Build history of the part. All positions in model axes, mm. Coordinates: 2 decimals unless noted, no trailing zeros. Order: outer loops, then holes, each group sorted by start corner. A loop starts at its lowest first (then second) coordinate and runs counter-clockwise, first axis right, second up. Notation, with made-up numbers: M 51.25,-25.75 L 57.25,-25.75 A21 cw 57.25,-12.75 Z; hole C -2,-15 d9. An arc over 180 degrees is marked long. Use a Markdown table: item, result. Add a question column.
from build123d import *

# Parameters (mm, degrees)
SKETCH1_R             = 5
BOSS_EXTRUDE1_DEPTH   = 10
BOSS_EXTRUDE1_2_DEPTH = 10
BOSS_EXTRUDE2_START   = 4
SKETCH1_3_W           = 162
SKETCH1_3_H           = 50
SKETCH1_3_W_2         = 154
SKETCH1_3_H_2         = 42
SKETCH1_3_R           = 5
BOSS_EXTRUDE2_DEPTH   = 4
SKETCH1_4_W           = 162
SKETCH1_4_H           = 50
SKETCH1_4_W_2         = 154
SKETCH1_4_H_2         = 42
BOSS_EXTRUDE3_DEPTH   = 96
FILLET1_R             = 4
SKETCH2_W             = 162
SKETCH2_H             = 50
SKETCH2_W_2           = 154
SKETCH2_H_2           = 42
BOSS_EXTRUDE4_DEPTH   = 5
SKETCH2_2_W           = 162
SKETCH2_2_H           = 50
SKETCH2_2_W_2         = 154
SKETCH2_2_H_2         = 42
BOSS_EXTRUDE5_DEPTH   = 5
SKETCH3_R             = 5
CUT_EXTRUDE1_DEPTH    = 10
SKETCH4_W             = 162
SKETCH4_H             = 50
BOSS_EXTRUDE6_DEPTH   = 10


with BuildPart() as part:
    # Sketch1 → Boss-Extrude1 (new body)
    with BuildSketch(Plane(origin=(0, 0, 0), x_dir=(1, 0, 0), z_dir=(0, 1, 0))):
        with Locations(Location((-57, 8.550438596, 0), (0, 0, 270))):
            Circle(SKETCH1_R)
    extrude(amount=-BOSS_EXTRUDE1_DEPTH)



with BuildPart() as body_2:
    # Sketch1 → Boss-Extrude1 2 (new body)
    with BuildSketch(Plane(origin=(0, 0, 0), x_dir=(1, 0, 0), z_dir=(0, 1, 0))):
        with Locations(Location((57, 8.550438596, 0), (0, 0, 270))):
            Circle(SKETCH1_R)
    extrude(amount=-BOSS_EXTRUDE1_2_DEPTH)


with BuildPart() as part_1:
    add(part.part)

    add(body_2.part)  # Boss-Extrude2 merges body 2
    # Sketch1_3 → Boss-Extrude2 (add)
    # profile 1 of 4: a face of its own
    with BuildSketch(Plane(origin=(0, 0, 0), x_dir=(1, 0, 0), z_dir=(0, 1, 0)).offset(BOSS_EXTRUDE2_START)):
        with Locations((0, 8.550438596)):
            Rectangle(SKETCH1_3_W, SKETCH1_3_H)
        with Locations((0, 8.550438596)):
            Rectangle(SKETCH1_3_W_2, SKETCH1_3_H_2, mode=Mode.SUBTRACT)
    # profile 2 of 4: a face of its own
    with BuildSketch(Plane(origin=(0, 0, 0), x_dir=(1, 0, 0), z_dir=(0, 1, 0)).offset(BOSS_EXTRUDE2_START)):
        with Locations((0, 8.550438596)):
            Rectangle(SKETCH1_3_W_2, SKETCH1_3_H_2)
        with Locations(Location((57, 8.550438596, 0), (0, 0, 270))):
            Circle(SKETCH1_3_R, mode=Mode.SUBTRACT)
        with Locations(Location((-57, 8.550438596, 0), (0, 0, 270))):
            Circle(SKETCH1_3_R, mode=Mode.SUBTRACT)
    # profile 3 of 4: a face of its own
    with BuildSketch(Plane(origin=(0, 0, 0), x_dir=(1, 0, 0), z_dir=(0, 1, 0)).offset(BOSS_EXTRUDE2_START)):
        with Locations(Location((-57, 8.550438596, 0), (0, 0, 270))):
            Circle(SKETCH1_3_R)
    # profile 4 of 4: a face of its own
    with BuildSketch(Plane(origin=(0, 0, 0), x_dir=(1, 0, 0), z_dir=(0, 1, 0)).offset(BOSS_EXTRUDE2_START)):
        with Locations(Location((57, 8.550438596, 0), (0, 0, 270))):
            Circle(SKETCH1_3_R)
    extrude(amount=-BOSS_EXTRUDE2_DEPTH)

    # Sketch1_4 → Boss-Extrude3 (add)
    with BuildSketch(Plane(origin=(0, 0, 0), x_dir=(1, 0, 0), z_dir=(0, 1, 0))):
        with Locations((0, 8.550438596)):
            Rectangle(SKETCH1_4_W, SKETCH1_4_H)
        with Locations((0, 8.550438596)):
            Rectangle(SKETCH1_4_W_2, SKETCH1_4_H_2, mode=Mode.SUBTRACT)
    extrude(amount=BOSS_EXTRUDE3_DEPTH)

    # Fillet1
    fillet1_edges = [part_1.edges().sort_by_distance(p)[0] for p in [
        (0, 0, 16.449561404),
        (81, 0, -8.550438596),
        (-81, 0, -8.550438596),
        (0, 0, -33.550438596),
    ]]
    fillet(fillet1_edges, radius=FILLET1_R)



with BuildPart() as body_2_2:
    # Sketch2 → Boss-Extrude4 (new body)
    with BuildSketch(Plane(origin=(0, 96, 0), x_dir=(1, 0, 0), z_dir=(0, 1, 0))):
        with Locations((0, 8.550438596)):
            Rectangle(SKETCH2_W, SKETCH2_H)
        with Locations((0, 8.550438596)):
            Rectangle(SKETCH2_W_2, SKETCH2_H_2, mode=Mode.SUBTRACT)
    extrude(amount=BOSS_EXTRUDE4_DEPTH)


with BuildPart() as part_2:
    add(part_1.part)

    add(body_2_2.part)  # Boss-Extrude5 merges body 2 2
    # Sketch2_2 → Boss-Extrude5 (add)
    with BuildSketch(Plane(origin=(0, 96, 0), x_dir=(1, 0, 0), z_dir=(0, 1, 0))):
        with Locations((0, 8.550438596)):
            Rectangle(SKETCH2_2_W, SKETCH2_2_H)
        with Locations((0, 8.550438596)):
            Rectangle(SKETCH2_2_W_2, SKETCH2_2_H_2, mode=Mode.SUBTRACT)
    extrude(amount=BOSS_EXTRUDE5_DEPTH)

    # Sketch3 → Cut-Extrude1 (cut)
    with BuildSketch(Plane(origin=(0, 0, -33.550438596), x_dir=(-1, 0, 0), z_dir=(0, 0, -1))):
        with Locations((0, 53.488312156)):
            Circle(SKETCH3_R)
    extrude(amount=-CUT_EXTRUDE1_DEPTH, mode=Mode.SUBTRACT)

    # Sketch4 → Boss-Extrude6 (add)
    with BuildSketch(Plane(origin=(0, 101, 0), x_dir=(1, 0, 0), z_dir=(0, 1, 0))):
        with Locations((0, 8.550438596)):
            Rectangle(SKETCH4_W, SKETCH4_H)
    extrude(amount=BOSS_EXTRUDE6_DEPTH)


solid = part_2.part
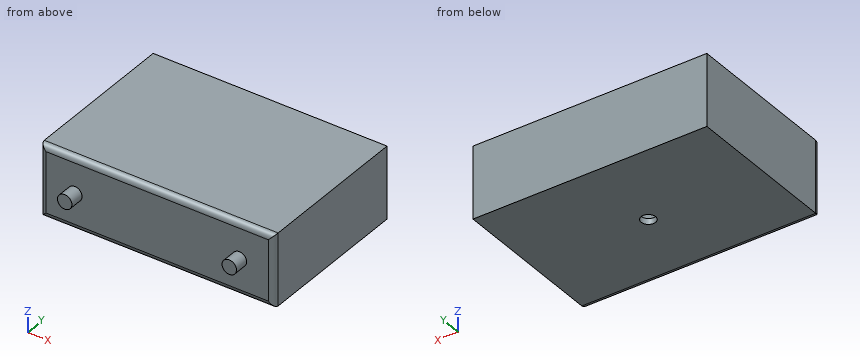
(1) Slice it at D-D on x = -57. Give the cut face in (y, z).
(2) Slice it at A-A on y = 71.5. Give the cut face in (x, z), and give its area (3 significant figures).
(3) Slice it at B-B on x = -11. Give the cut face in (y, z).
(4) Slice it at C-C on z = 8. Give the cut face in (x, y), and give its area (3 significant figures).
(5) Drill centre lines: line 1 along X through (y, z) = (69, -14); line 2 along Y through (x, z) = (13.5, -13.5); line 3 along Z through (x, y) = (-44.5, 47). Where is each one in solid material? Low to high. Write a range as from..to.
(6) Drop a flat-ended pin along its axis: P1, Ø10, axis at x = -18.5, z = -20.5, coming from the -Y side. Give the stop position or say it passes through.
Solutions:
| question | item | result |
|---|---|---|
| 1 | outline | M -10,-13.55 L 0,-13.55 L 0,-29.55 A4 ccw 4,-33.55 L 111,-33.55 L 111,16.45 L 4,16.45 A4 ccw 0,12.45 L 0,-3.55 L -10,-3.55 Z; hole M 4,-29.55 L 101,-29.55 L 101,12.45 L 4,12.45 Z |
| 2 | outline | M -81,-33.55 L 81,-33.55 L 81,16.45 L -81,16.45 Z; hole M -77,-29.55 L 77,-29.55 L 77,12.45 L -77,12.45 Z |
| 2 | area | 1,630 mm² |
| 3 | outline | M 0,-29.55 A4 ccw 4,-33.55 L 111,-33.55 L 111,16.45 L 4,16.45 A4 ccw 0,12.45 Z; hole M 4,-29.55 L 101,-29.55 L 101,12.45 L 4,12.45 Z |
| 4 | outline | M -81,4 A4 ccw -77,0 L 77,0 A4 ccw 81,4 L 81,111 L -81,111 Z; hole M -77,4 L 77,4 L 77,101 L -77,101 Z |
| 4 | area | 3,040 mm² |
| 5 | line 1 | -81..-77, 77..81 |
| 5 | line 2 | 0..4, 101..111 |
| 5 | line 3 | -33.55..-29.55, 12.45..16.45 |
| 6 | P1 | y = 0 |
